from build123d import *

# Parameters (mm, degrees)
F1_DEPTH  = 13
F2_R      = 6.8523627272
F3_DEPTH  = 30
F4_DEPTH  = 20
F5_W      = 25.9563405998
F5_H      = 14
F6_DEPTH  = 15
F7_W      = 24.6814545244
F7_H      = 12.1941640973
F8_DEPTH  = 14
F9_R      = 5.0327145122
F9_R_2    = 4.9558235457
F10_DEPTH = 3
F11_W     = 25.9563405998
F11_H     = 14
F12_DEPTH = 3
F13_R     = 4.05
F14_DEPTH = 5


with BuildPart() as f1:
    # F0 (on Front) → F1 (new body)
    with BuildSketch(Plane.XZ):
        with BuildLine():
            ThreePointArc((-21.9452433995, 6.3125732282), (-30.7452433995, 9.5621885901), (-21.9452433995, 12.8118039519))
            ThreePointArc((-21.9452433995, 12.8118039519), (-21.4056409565, 13.6804284443), (-20.7452433995, 14.4611680756))
            ThreePointArc((-20.7452433995, 14.4611680756), (-23.0334963979, 16.0155929784), (-25.7452433995, 16.5621885901))
            ThreePointArc((-25.7452433995, 16.5621885901), (-32.7452433995, 9.5621885901), (-25.7452433995, 2.5621885901))
            ThreePointArc((-25.7452433995, 2.5621885901), (-23.0334963979, 3.1087842017), (-20.7452433995, 4.6632091045))
            ThreePointArc((-20.7452433995, 4.6632091045), (-21.4056409565, 5.4439487359), (-21.9452433995, 6.3125732282))
        make_face()
        with BuildLine():
            ThreePointArc((-20.7452433995, 14.4611680756), (-20.0848458425, 13.6804284443), (-19.5452433995, 12.8118039519))
            ThreePointArc((-19.5452433995, 12.8118039519), (-14.0131925919, 14.2526043499), (-10.7452433995, 9.5621885901))
            ThreePointArc((-10.7452433995, 9.5621885901), (-14.0131925919, 4.8717728303), (-19.5452433995, 6.3125732282))
            ThreePointArc((-19.5452433995, 6.3125732282), (-20.0848458425, 5.4439487359), (-20.7452433995, 4.6632091045))
            ThreePointArc((-20.7452433995, 4.6632091045), (-18.4569904011, 3.1087842017), (-15.7452433995, 2.5621885901))
            ThreePointArc((-15.7452433995, 2.5621885901), (-10.7954959312, 4.6124411218), (-8.7452433995, 9.5621885901))
            ThreePointArc((-8.7452433995, 9.5621885901), (-10.7954959312, 14.5119360584), (-15.7452433995, 16.5621885901))
            ThreePointArc((-15.7452433995, 16.5621885901), (-18.4569904011, 16.0155929784), (-20.7452433995, 14.4611680756))
        make_face()
        with BuildLine():
            ThreePointArc((-25.7452433995, 16.5621885901), (-23.0334963979, 16.0155929784), (-20.7452433995, 14.4611680756))
            ThreePointArc((-20.7452433995, 14.4611680756), (-18.4569904011, 16.0155929784), (-15.7452433995, 16.5621885901))
            Line((-15.7452433995, 16.5621885901), (-25.7452433995, 16.5621885901))
        make_face()
        with BuildLine():
            ThreePointArc((-15.7452433995, 2.5621885901), (-18.4569904011, 3.1087842017), (-20.7452433995, 4.6632091045))
            ThreePointArc((-20.7452433995, 4.6632091045), (-23.0334963979, 3.1087842017), (-25.7452433995, 2.5621885901))
            Line((-25.7452433995, 2.5621885901), (-15.7452433995, 2.5621885901))
        make_face()
    extrude(amount=F1_DEPTH)

    # F2 (on face) → F3 (cut)
    with BuildSketch(Plane.XZ.offset(13)):
        with Locations((-20.7452433995, 9.5621885901)):
            Circle(F2_R)
    extrude(amount=-F3_DEPTH, mode=Mode.SUBTRACT)

    # F0 (on Front) → F4 (join)
    with BuildSketch(Plane.XZ):
        with BuildLine():
            ThreePointArc((-21.9452433995, 6.3125732282), (-21.0548276397, 7.8301377825), (-20.7452433995, 9.5621885901))
            ThreePointArc((-20.7452433995, 9.5621885901), (-21.0548276397, 11.2942393976), (-21.9452433995, 12.8118039519))
            ThreePointArc((-21.9452433995, 12.8118039519), (-22.7452433995, 9.5621885901), (-21.9452433995, 6.3125732282))
        make_face()
        with BuildLine():
            ThreePointArc((-19.5452433995, 6.3125732282), (-20.4356591593, 7.8301377825), (-20.7452433995, 9.5621885901))
            ThreePointArc((-20.7452433995, 9.5621885901), (-21.0548276397, 7.8301377825), (-21.9452433995, 6.3125732282))
            ThreePointArc((-21.9452433995, 6.3125732282), (-21.4056409565, 5.4439487359), (-20.7452433995, 4.6632091045))
            ThreePointArc((-20.7452433995, 4.6632091045), (-20.0848458425, 5.4439487359), (-19.5452433995, 6.3125732282))
        make_face()
        with BuildLine():
            ThreePointArc((-21.9452433995, 12.8118039519), (-21.0548276397, 11.2942393976), (-20.7452433995, 9.5621885901))
            ThreePointArc((-20.7452433995, 9.5621885901), (-20.4356591593, 11.2942393976), (-19.5452433995, 12.8118039519))
            ThreePointArc((-19.5452433995, 12.8118039519), (-20.0848458425, 13.6804284443), (-20.7452433995, 14.4611680756))
            ThreePointArc((-20.7452433995, 14.4611680756), (-21.4056409565, 13.6804284443), (-21.9452433995, 12.8118039519))
        make_face()
        with BuildLine():
            ThreePointArc((-19.5452433995, 12.8118039519), (-20.4356591593, 11.2942393976), (-20.7452433995, 9.5621885901))
            ThreePointArc((-20.7452433995, 9.5621885901), (-20.4356591593, 7.8301377825), (-19.5452433995, 6.3125732282))
            ThreePointArc((-19.5452433995, 6.3125732282), (-18.9481852123, 7.888868537), (-18.7452433995, 9.5621885901))
            ThreePointArc((-18.7452433995, 9.5621885901), (-18.9481852123, 11.2355086431), (-19.5452433995, 12.8118039519))
        make_face()
        with BuildLine():
            ThreePointArc((-21.9452433995, 6.3125732282), (-30.7452433995, 9.5621885901), (-21.9452433995, 12.8118039519))
            ThreePointArc((-21.9452433995, 12.8118039519), (-21.4056409565, 13.6804284443), (-20.7452433995, 14.4611680756))
            ThreePointArc((-20.7452433995, 14.4611680756), (-23.0334963979, 16.0155929784), (-25.7452433995, 16.5621885901))
            ThreePointArc((-25.7452433995, 16.5621885901), (-32.7452433995, 9.5621885901), (-25.7452433995, 2.5621885901))
            ThreePointArc((-25.7452433995, 2.5621885901), (-23.0334963979, 3.1087842017), (-20.7452433995, 4.6632091045))
            ThreePointArc((-20.7452433995, 4.6632091045), (-21.4056409565, 5.4439487359), (-21.9452433995, 6.3125732282))
        make_face()
        with BuildLine():
            ThreePointArc((-20.7452433995, 14.4611680756), (-20.0848458425, 13.6804284443), (-19.5452433995, 12.8118039519))
            ThreePointArc((-19.5452433995, 12.8118039519), (-14.0131925919, 14.2526043499), (-10.7452433995, 9.5621885901))
            ThreePointArc((-10.7452433995, 9.5621885901), (-14.0131925919, 4.8717728303), (-19.5452433995, 6.3125732282))
            ThreePointArc((-19.5452433995, 6.3125732282), (-20.0848458425, 5.4439487359), (-20.7452433995, 4.6632091045))
            ThreePointArc((-20.7452433995, 4.6632091045), (-18.4569904011, 3.1087842017), (-15.7452433995, 2.5621885901))
            ThreePointArc((-15.7452433995, 2.5621885901), (-10.7954959312, 4.6124411218), (-8.7452433995, 9.5621885901))
            ThreePointArc((-8.7452433995, 9.5621885901), (-10.7954959312, 14.5119360584), (-15.7452433995, 16.5621885901))
            ThreePointArc((-15.7452433995, 16.5621885901), (-18.4569904011, 16.0155929784), (-20.7452433995, 14.4611680756))
        make_face()
        with BuildLine():
            ThreePointArc((-25.7452433995, 16.5621885901), (-23.0334963979, 16.0155929784), (-20.7452433995, 14.4611680756))
            ThreePointArc((-20.7452433995, 14.4611680756), (-18.4569904011, 16.0155929784), (-15.7452433995, 16.5621885901))
            Line((-15.7452433995, 16.5621885901), (-25.7452433995, 16.5621885901))
        make_face()
        with BuildLine():
            ThreePointArc((-15.7452433995, 2.5621885901), (-18.4569904011, 3.1087842017), (-20.7452433995, 4.6632091045))
            ThreePointArc((-20.7452433995, 4.6632091045), (-23.0334963979, 3.1087842017), (-25.7452433995, 2.5621885901))
            Line((-25.7452433995, 2.5621885901), (-15.7452433995, 2.5621885901))
        make_face()
    extrude(amount=F4_DEPTH)

    # F5 (on face) → F6 (join)
    with BuildSketch(Plane.XZ.offset(20)):
        with Locations((-20.5991824623, 9.5621885901)):
            Rectangle(F5_W, F5_H)
    extrude(amount=F6_DEPTH)

    # F7 (on face) → F8 (cut)
    with BuildSketch(Plane.XZ.offset(35)):
        with Locations((-20.5570058897, 9.6122492105)):
            Rectangle(F7_W, F7_H)
    extrude(amount=-F8_DEPTH, mode=Mode.SUBTRACT)

    # F9 (on face) → F10 (cut)
    with BuildSketch(Plane.XZ.offset(21)):
        with Locations((-25.7452465594, 9.5622381195)):
            Circle(F9_R)
        with Locations((-15.7452113926, 9.5622753724)):
            Circle(F9_R_2)
    extrude(amount=-F10_DEPTH, mode=Mode.SUBTRACT)

    # F11 (on face) → F12 (join)
    with BuildSketch(Plane.XZ.offset(35)):
        with Locations((-20.5991824623, 9.5621885901)):
            Rectangle(F11_W, F11_H)
    extrude(amount=F12_DEPTH)

    # F13 (on face) → F14 (cut)
    with BuildSketch(Plane.XZ.offset(38)):
        with Locations((-20.5991824623, 9.5770442858)):
            Circle(F13_R)
    extrude(amount=-F14_DEPTH, mode=Mode.SUBTRACT)


solid = f1.part
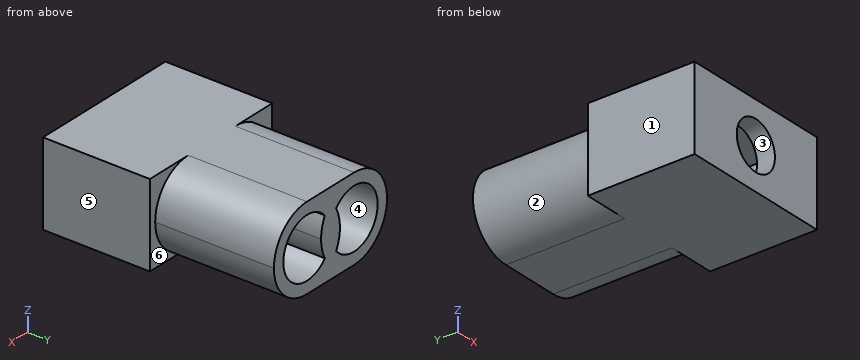
Design review of the part built by this model. Coordinates are the model's own, in mm. Face numbers are marked on the shaded views. A direction names the side the tool comes from. Coordinates: 2 decimals unless noted, no trailing zeros. Order: outer loops, then holes, each group sorted by start corner. A loop starts at its lowest first (then second) coordinate and runs counter-clockwise, first axis right, second up.
Item 1: For line 1 (Y direction, x = -29.5, z = 14); line 2 (Z direction, x = -10, y = -31); line 3 (X direction, y = -10, z = 6), list the stretches that pass through material, from the lowest coordinate up.
Item 2: Take a section at D-D, the plane z = 6.75. Count the separate pieces of the cut face and the enclosed holes in it, then the cut area to 3 significant figures.
Item 3: Take a section at A-A, the plane y = -14. Write out the cut boundary in (x, z).
Item 4: For pin 1 Ø2.5 at (x, z) = (-13, 9) entering from +Y; pin 2 Ø8 at (y, z) = (-9.5, 8) entering from -X; pin 3 Ø2 at (x, z) = (-19.5, 11) entering from -Y, all flat-tipped, find the tip position at first contact; note any pin that passes through.
Item 5: Take a section at C-C, the plane y = -24.5. Write out the cut boundary in (x, z).
Item 6: For the marked faces 1, 2 and 3, list the 3-axis set-ups (+Z, -Z, +X, -X, +Y, -Y) from which the entire face can be reached by the end or side of a thin tool; tool diameter is ignored.
Item 7: The part is to be moulded in two halves that separate along X. For the marked faces 4, 5 and 6, say which applies: pulls with the +X half, pulls with the -X half, needs draft (parallel to the pull), parting line crosses it, or undercut.
Item 8: Take a section at B-B, the plane x = -17.5. Write out the cut boundary in (y, z).
The answers:
1. line 1: y = -38 to -35, -21 to 0
1. line 2: z = 2.56 to 3.52, 15.71 to 16.56
1. line 3: x = -31.77 to -29.25, -22.24 to -19.25, -12.24 to -9.72
2. separate pieces: 3
2. enclosed holes: 0
2. area: 233 mm2
3. outline: (-25.75, 2.56) - (-15.75, 2.56) arc R7 ccw to (-15.75, 16.56) - (-25.75, 16.56) arc R7 ccw to start; hole (-21.95, 6.31) arc R7 cw to (-21.95, 12.81) arc R5 ccw (long way) to start; hole (-19.55, 6.31) arc R5 ccw (long way) to (-19.55, 12.81) arc R7 cw to start
4. pin 1: stops at y = -35
4. pin 2: stops at x = -32.75
4. pin 3: stops at y = -21
5. outline: (-33.58, 2.56) - (-7.62, 2.56) - (-7.62, 16.56) - (-33.58, 16.56) - close; hole (-32.9, 3.52) - (-8.22, 3.52) - (-8.22, 15.71) - (-32.9, 15.71) - close
6. face 1: +Z, -Z, -X, +Y, -Y
6. face 2: -X, +Y
6. face 3: -Y
7. face 4: undercut
7. face 5: pulls with the +X half
7. face 6: needs draft
8. outline: (-38, 2.56) - (0, 2.56) - (0, 4.88) - (-20, 4.88) - (-20, 4.93) - (-21, 4.93) - (-21, 3.52) - (-35, 3.52) - (-35, 6.97) - (-38, 6.97) - close; (-38, 12.18) - (-35, 12.18) - (-35, 15.71) - (-21, 15.71) - (-21, 14.2) - (-20, 14.2) - (-20, 14.24) - (0, 14.24) - (0, 16.56) - (-38, 16.56) - close
